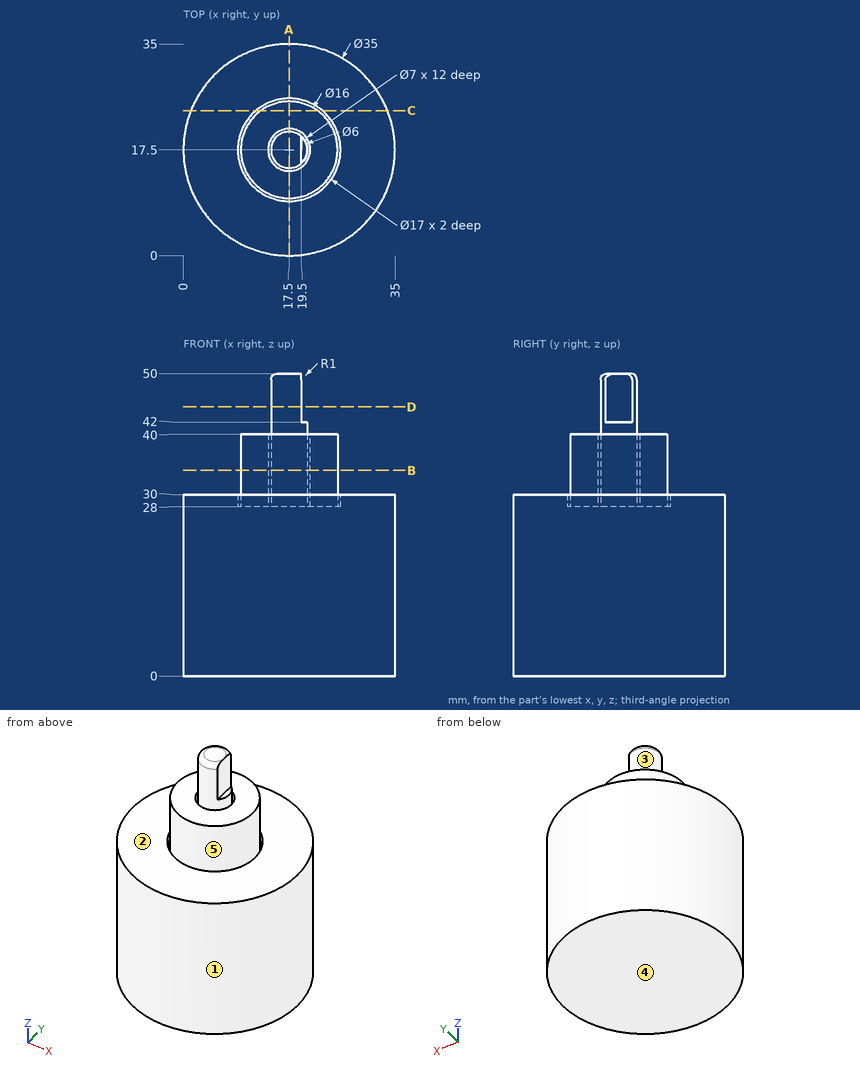
Here's the drawing with two shaded views (mm, measured from the low corner). I have some questions. A direction names the side the tool comes from. Round coordinates to 2 decimals unless told otherwise and drop trailing zeros. Loops run counter-clockwise (first coordinate to the right, second up) from the corner with the lowest first, then second, coordinate; pieces in that order, holes last. Notation, with made-up numbers: M 60.25,21.5 L 118.25,21.5 A24 ccw 118.25,34.5 Z; hole C 87,-18 d9. An arc over 180 degrees is marked long. Answer as CSV lines item,"result".
1) Which directions (+Z, -Z, +X, -X, +Y, -Y) give clear straight access to the entire face, cutting with the end or side of a thin tool? Please do the marked faces 4 and 5.
From the geometry:
face 4,"-Z, +X, -X, +Y, -Y"
face 5,"+Z"
2) We'd pull the mould along X, two halves only. Please class the marked faces 1, 2 and 3: released by +X, released by -X, zero draft, split by the parting line, or undercut.
From the geometry:
face 1,"split by the parting line"
face 2,"zero draft"
face 3,"undercut"
3) If I drill on probe 1 along Y at (x, z) = (17.5, 28.6); probe 2 along Y at (x, z) = (17.5, 35.75); probe 3 along Z at (x, y) = (7.5, 7), over which ranges is the centre line in solid material (lowest first)?
From the geometry:
probe 1,"0 to 9, 9.5 to 14, 14.5 to 20.5, 21 to 25.5, 26 to 35"
probe 2,"9.5 to 14, 14.5 to 20.5, 21 to 25.5"
probe 3,"0 to 30"
4) Imagine slicing it at A-A on x = 17.5. List the corners of the cut face in (y, z) for me.
From the geometry:
outline,"M 0,0 L 35,0 L 35,30 L 26,30 L 26,28 L 25.5,28 L 25.5,40 L 21,40 L 21,28 L 20.5,28 L 20.5,49 A1 ccw 19.5,50 L 15.5,50 A1 ccw 14.5,49 L 14.5,28 L 14,28 L 14,40 L 9.5,40 L 9.5,28 L 9,28 L 9,30 L 0,30 Z"
5) Imagine slicing it at B-B on z = 34. List the corners of the cut face in (x, y) for me, and give its area (3 significant figures).
From the geometry:
outline,"C 17.5,17.5 d16; C 17.5,17.5 d6; hole C 17.5,17.5 d7"
area,"191 mm^2"
6) Imagine slicing it at C-C on y = 24. List the corners of the cut face in (x, z) for me.
From the geometry:
outline,"M 1.25,0 L 33.75,0 L 33.75,30 L 22.98,30 L 22.98,28 L 22.16,28 L 22.16,40 L 12.84,40 L 12.84,28 L 12.02,28 L 12.02,30 L 1.25,30 Z"
7) For pin 1 Ø15.5 at (x, y) = (17.5, 17.5) entering from -Z; pin 2 Ø6 at (x, z) = (26.5, 7.5) entering from +Y; pin 3 Ø1 at (y, z) = (15.5, 29) entering from +X; pin 4 Ø0.8 at (x, y) = (20, 16.5) entering from +Z, each with a flat end and sliding along its axis, tell me the tip position at first contact or that it passes through.
From the geometry:
pin 1,"z = 0"
pin 2,"y = 33.94"
pin 3,"x = 34.94"
pin 4,"z = 42"
8) Imagine slicing it at D-D on z = 44.5. List the corners of the cut face in (x, y) for me.
From the geometry:
outline,"M 19.5,15.26 L 19.5,19.74 A3 ccw long Z"
